Autodesk Inventor part; units mm, degrees
ref_plane "YZ Plane" through (0, 0, 0) normal (1, 0, 0) x (0, 1, 0)
ref_plane "XZ Plane" through (0, 0, 0) normal (0, 1, 0) x (-1, 0, 0)
ref_plane "XY Plane" through (0, 0, 0) normal (0, 0, 1) x (1, 0, 0)
sketch "Skizze1" plane through (0, 0, 0) normal (0, 0, 1) x (1, 0, 0)
  line L0 (-188.78, 10) -> (188.78, 10)
  line L1 (188.78, 10) -> (188.78, -10)
  line L2 (188.78, -10) -> (-188.78, -10)
  line L3 (-188.78, -10) -> (-188.78, 10)
  line L4 (0, -14) -> (0, 14) construction
  line L5 (-264.292, 0) -> (264.292, 0) construction
  point P0 (0, 0)
  dimension "d0" = 377.56
  dimension "d1" = 20
extrude "Extrusion1" add sketch "Skizze1" along normal blind 2
sketch "Skizze3" plane through (0, 0, 2) normal (0, 0, 1) x (1, 0, 0)
  circle A0 centre (-184.78, 0) radius 1.5
  line L0 (-188.78, 10) -> (-188.78, -10)
  line L1 (-264.292, 0) -> (264.292, 0)
  circle A1 centre (-93.64, 6) radius 1.5
  line L2 (188.78, 10) -> (-188.78, 10)
  line L3 (0, -14) -> (0, 14)
  point P0 (0, 0)
  dimension "d8" = 3
  dimension "d9" = 4
  dimension "d10" = 3
  dimension "d11" = 4
  dimension "d12" = 95.14
  dimension "d13" = 93.64
extrude "Extrusion3" cut sketch "Skizze3" against normal through all contours L1 A0 | A0 L1 | A1
mirror "Spiegeln2" about plane through (0, 0, 0) normal (1, 0, 0) of "Extrusion3"
sketch "Skizze4" plane through (0, 0, 0) normal (0, 0, -1) x (-1, 0, 0)
  line L0 (187.28, 8.2503) -> (187.28, 3.5)
  line L1 (187.28, 3.5) -> (185.78, 3.5)
  line L2 (185.78, 3.5) -> (185.78, 7)
  line L3 (185.78, 7) -> (182.28, 7)
  line L4 (182.28, 7) -> (182.28, 8.5)
  line L5 (182.28, 8.5) -> (187.28, 8.5)
  line L6 (187.28, 8.5) -> (187.28, 8.2503)
  line L7 (188.78, 10) -> (188.78, -10)
  line L8 (-188.78, 10) -> (188.78, 10)
  point P0 (0, 0)
  dimension "d16" = 1.5
  dimension "d17" = 1.5
  dimension "d18" = 1.5
  dimension "d19" = 1.5
  dimension "d20" = 5
  dimension "d21" = 5
extrude "Extrusion4" add sketch "Skizze4" along normal blind 1
mirror "Spiegeln3" about plane through (0, 0, 0) normal (1, 0, 0) of "Extrusion4"
mirror "Spiegeln5" about plane through (0, 0, 0) normal (0, 1, 0) of "Extrusion4", "Spiegeln3"
sketch "Skizze5" plane through (-182.28, -8.5, -1) normal (0, 0, -1) x (-1, 0, 0)
  line L0 (0, 1.5) -> (3.5, 1.5)
  line L1 (5, 0) -> (0, 0)
  line L2 (3.5, 1.5) -> (0, 1.5)
  line L3 (0, 1.5) -> (0, 0)
  line L4 (0, 0) -> (3.5, 0)
  line L5 (3.5, 0) -> (3.5, 1.5)
  point P0 (-182.28, 8.5)
extrude "Extrusion5" cut sketch "Skizze5" against normal blind 1
properties part number "PCB_Kabelkanaldeckel_1.0"
Check sheet for the modelled part. Datum: model origin and axes. Units: mm. Round coordinates to 2 decimals unless told otherwise and drop trailing zeros. Order: outer loops, then holes, each group sorted by start corner. A loop starts at its lowest first (then second) coordinate and runs counter-clockwise, first axis right, second up. Notation, with made-up numbers: (25, 30) - (76, 30) arc R26 cw to (76, 49) - close; hole circle Ø1 at (89.5, -24). An arc over 180 degrees is marked (long way). Write item = value, one per line.
Q1. Draft check along X on faces 1 (the face through (-3, 0, 0)), 2 (the face through (-3, 0, 2)). Enter one of: pulls with the +X half, pulls with the -X half, needs draft (parallel to the pull), parting line crosses it, or undercut.
Computed:
face_1 = undercut
face_2 = needs draft
Q2. Go/stop test with flat-tipped pins: pin 1 (2.5 mm diameter, centred on x = -184.78, y = 0, fed in from +Z); pin 2 (0.8 mm diameter, centred on y = 5, z = -0.5, fed in from +X); pin 3 (3 mm diameter, centred on x = 73.5, y = -4, fed in from -Z); pin 4 (0.8 mm diameter, centred on x = 183.5, z = -0.5, fed in from +Y). Record where each tip stops, or that it passes through.
Computed:
pin_1 = through
pin_2 = 187.28
pin_3 = 0
pin_4 = 8.5
Q3. Section check A-A (x = 23.5). Record the boundary of the cut face in (y, z), and give its area (3 significant figures).
Computed:
outline = (-10, 0) - (10, 0) - (10, 2) - (-10, 2) - close
area = 40.0 mm^2
Q4. Thickness scan on line 1 along X through (y, z) = (0, 0.95); line 2 along X through (y, z) = (8, -0.55); line 3 along X through (y, z) = (1.25, 1.1). Record the ranges inside material, lowest first.
Computed:
line_1 = -188.78 to -186.28, -183.28 to 183.28, 186.28 to 188.78
line_2 = -187.28 to -182.28, 182.28 to 187.28
line_3 = -188.78 to -185.61, -183.95 to 183.95, 185.61 to 188.78
